Design review of the part built by this model. Coordinates are the model's own, in mm. Face numbers are marked on the shaded views. Give positions to 0.01 mm unless a question says otherwise; leave off trailing zeros. Loops run counter-clockwise (first coordinate to the right, second up) from the corner with the lowest first, then second, coordinate; pieces in that order, holes last. Notation, with made-up numbers: (-24.75, 72.5) - (2.25, 72.5) arc R20 cw to (2.25, 102.5) - close; hole circle Ø2 at (-40, -9.5). An arc over 180 degrees is marked (long way). Put each result on its own line as item: value. Start each with the question number.
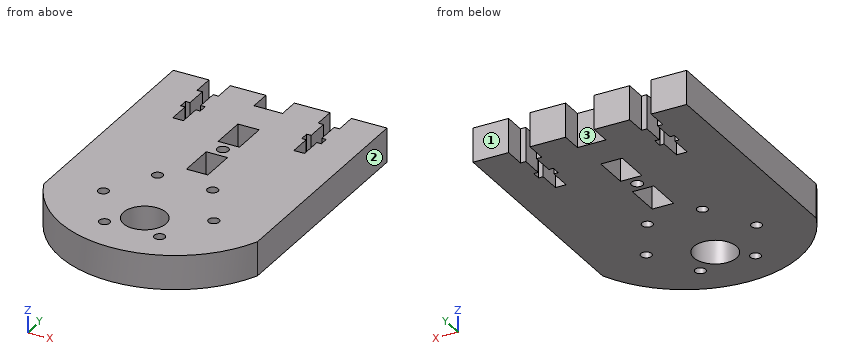
Autodesk Inventor part; units mm, degrees
ref_plane "YZ Plane" through (0, 0, 0) normal (1, 0, 0) x (0, 1, 0)
ref_plane "XZ Plane" through (0, 0, 0) normal (0, 1, 0) x (-1, 0, 0)
ref_plane "XY Plane" through (0, 0, 0) normal (0, 0, 1) x (1, 0, 0)
sketch "0" plane through (0, 0, 0) normal (0, 0, 1) x (1, 0, 0)
  line L0 (4.1594, 49.6005) -> (4.1594, 55.8505)
  line L1 (4.1594, 55.8505) -> (14.5761, 55.8505)
  line L2 (14.5761, 55.8505) -> (14.5761, 49.6005)
  line L3 (20.8261, 49.6005) -> (19.2636, 49.6005)
  line L4 (19.2636, 49.6005) -> (19.2636, 43.09)
  line L5 (19.2636, 33.9755) -> (16.1386, 33.9755)
  line L6 (16.1386, 33.9755) -> (16.1386, 40.4859)
  line L7 (14.8365, 43.09) -> (16.1386, 43.09)
  line L8 (20.5657, 43.09) -> (20.5657, 40.4859)
  line L9 (20.5657, 40.4859) -> (19.2636, 40.4859)
  line L10 (14.8365, 40.4859) -> (14.8365, 43.09)
  line L11 (16.1386, 43.09) -> (16.1386, 49.6005)
  line L12 (16.1386, 40.4859) -> (14.8365, 40.4859)
  line L13 (19.2636, 43.09) -> (20.5657, 43.09)
  line L14 (16.1386, 49.6005) -> (14.5761, 49.6005)
  line L15 (20.8261, 55.8505) -> (31.2428, 55.8505)
  line L16 (20.8261, 49.6005) -> (20.8261, 55.8505)
  line L17 (31.2428, 55.8505) -> (31.2428, 49.6005)
  line L18 (19.2636, 40.4859) -> (19.2636, 33.9755)
  line L19 (-31.2572, 49.6005) -> (-31.2572, 55.8505)
  line L20 (-31.2572, 55.8505) -> (-20.8406, 55.8505)
  line L21 (-14.5906, 55.8505) -> (-4.1739, 55.8505)
  line L22 (-4.1739, 55.8505) -> (-4.1739, 49.6005)
  line L23 (-3.1322, 49.6005) -> (-4.1739, 49.6005)
  line L24 (3.1178, 49.6005) -> (4.1594, 49.6005)
  line L25 (-20.8406, 55.8505) -> (-20.8406, 49.6005)
  line L26 (-14.5906, 49.6005) -> (-16.1531, 49.6005)
  line L27 (-16.1531, 49.6005) -> (-16.1531, 43.09)
  line L28 (-16.1531, 33.9755) -> (-19.2781, 33.9755)
  line L29 (-19.2781, 33.9755) -> (-19.2781, 40.4859)
  line L30 (-20.5802, 43.09) -> (-19.2781, 43.09)
  line L31 (-14.851, 43.09) -> (-14.851, 40.4859)
  line L32 (-14.851, 40.4859) -> (-16.1531, 40.4859)
  line L33 (-20.5802, 40.4859) -> (-20.5802, 43.09)
  line L34 (-19.2781, 43.09) -> (-19.2781, 49.6005)
  line L35 (-19.2781, 40.4859) -> (-20.5802, 40.4859)
  line L36 (-16.1531, 43.09) -> (-14.851, 43.09)
  line L37 (-19.2781, 49.6005) -> (-20.8406, 49.6005)
  line L38 (-14.5906, 49.6005) -> (-14.5906, 55.8505)
  line L39 (-16.1531, 40.4859) -> (-16.1531, 33.9755)
  arc A0 (-31.2572, -12.3787) -> (31.2428, -12.3787) centre (-0.0072, 0.6421) ccw
  circle A1 centre (8.0657, 5.7707) radius 1.5625
  circle A2 centre (-8.0802, 5.7707) radius 1.5625
  circle A3 centre (-16.1531, -8.212) radius 1.5625
  circle A4 centre (-8.0802, -22.1948) radius 1.5625
  circle A5 centre (8.0657, -22.1948) radius 1.5625
  circle A6 centre (16.1386, -8.212) radius 1.5625
  circle A7 centre (-0.0072, -15.5037) radius 6.25
  line L40 (31.2428, 49.6005) -> (31.2428, -12.3787)
  line L41 (-31.2572, -12.3787) -> (-31.2572, 49.6005)
  line L42 (-3.1322, 12.1005) -> (-3.1322, 22.5171)
  line L43 (-3.1322, 22.5171) -> (3.1178, 22.5171)
  line L44 (3.1178, 22.5171) -> (3.1178, 12.1005)
  line L45 (3.1178, 12.1005) -> (-3.1322, 12.1005)
  line L46 (-3.1322, 28.7671) -> (-3.1322, 39.1838)
  line L47 (3.1178, 39.1838) -> (3.1178, 28.7671)
  line L48 (3.1178, 28.7671) -> (-3.1322, 28.7671)
  circle A8 centre (-0.0072, 25.6421) radius 1.6667
  line L49 (-3.1322, 39.1838) -> (3.1178, 39.1838)
  line L50 (-3.1322, 49.6005) -> (3.1178, 49.6005)
  dimension "d0" = 12.5
sketch "Эскиз3" plane through (0, 0, 0) normal (0, 0, 1) x (1, 0, 0)
  circle A0 centre (-0.0072, -15.5037) radius 6.25
  circle A1 centre (-16.1531, -8.212) radius 1.5625
  circle A2 centre (-8.0802, 5.7707) radius 1.5625
  circle A3 centre (8.0657, 5.7707) radius 1.5625
  circle A4 centre (16.1386, -8.212) radius 1.5625
  circle A5 centre (8.0657, -22.1948) radius 1.5625
  circle A6 centre (-8.0802, -22.1948) radius 1.5625
  arc A7 (-31.2572, -12.3787) -> (31.2428, -12.3787) centre (-0.0072, 0.6421) ccw
  line L0 (-31.2572, -12.3787) -> (-31.2572, 49.6005)
  line L1 (-31.2572, 49.6005) -> (-31.2572, 55.8505)
  line L2 (-31.2572, 55.8505) -> (-20.8406, 55.8505)
  line L3 (-20.8406, 55.8505) -> (-20.8406, 49.6005)
  line L4 (-19.2781, 49.6005) -> (-20.8406, 49.6005)
  line L5 (-19.2781, 43.09) -> (-19.2781, 49.6005)
  line L6 (-20.5802, 43.09) -> (-19.2781, 43.09)
  line L7 (-20.5802, 40.4859) -> (-20.5802, 43.09)
  line L8 (-19.2781, 40.4859) -> (-20.5802, 40.4859)
  line L9 (-19.2781, 33.9755) -> (-19.2781, 40.4859)
  line L10 (-16.1531, 33.9755) -> (-19.2781, 33.9755)
  line L11 (-16.1531, 40.4859) -> (-16.1531, 33.9755)
  line L12 (-14.851, 40.4859) -> (-16.1531, 40.4859)
  line L13 (-14.851, 43.09) -> (-14.851, 40.4859)
  line L14 (-16.1531, 43.09) -> (-14.851, 43.09)
  line L15 (-16.1531, 49.6005) -> (-16.1531, 43.09)
  line L16 (-14.5906, 49.6005) -> (-16.1531, 49.6005)
  line L17 (-14.5906, 49.6005) -> (-14.5906, 55.8505)
  line L18 (-14.5906, 55.8505) -> (-4.1739, 55.8505)
  line L19 (-4.1739, 55.8505) -> (-4.1739, 49.6005)
  line L20 (-3.1322, 49.6005) -> (3.1178, 49.6005)
  line L21 (3.1178, 49.6005) -> (4.1594, 49.6005)
  line L22 (-3.1322, 49.6005) -> (-4.1739, 49.6005)
  line L23 (4.1594, 49.6005) -> (4.1594, 55.8505)
  line L24 (4.1594, 55.8505) -> (14.5761, 55.8505)
  line L25 (14.5761, 55.8505) -> (14.5761, 49.6005)
  line L26 (16.1386, 49.6005) -> (14.5761, 49.6005)
  line L27 (16.1386, 43.09) -> (16.1386, 49.6005)
  line L28 (14.8365, 43.09) -> (16.1386, 43.09)
  line L29 (14.8365, 40.4859) -> (14.8365, 43.09)
  line L30 (16.1386, 40.4859) -> (14.8365, 40.4859)
  line L31 (16.1386, 33.9755) -> (16.1386, 40.4859)
  line L32 (19.2636, 33.9755) -> (16.1386, 33.9755)
  line L33 (19.2636, 40.4859) -> (19.2636, 33.9755)
  line L34 (20.5657, 40.4859) -> (19.2636, 40.4859)
  line L35 (20.5657, 43.09) -> (20.5657, 40.4859)
  line L36 (19.2636, 43.09) -> (20.5657, 43.09)
  line L37 (19.2636, 49.6005) -> (19.2636, 43.09)
  line L38 (20.8261, 49.6005) -> (19.2636, 49.6005)
  line L39 (20.8261, 49.6005) -> (20.8261, 55.8505)
  line L40 (20.8261, 55.8505) -> (31.2428, 55.8505)
  line L41 (31.2428, 49.6005) -> (31.2428, -12.3787)
  line L42 (3.1178, 22.5171) -> (3.1178, 12.1005)
  circle A8 centre (-0.0072, 25.6421) radius 1.6667
  line L43 (3.1178, 28.7671) -> (-3.1322, 28.7671)
  line L44 (-3.1322, 28.7671) -> (-3.1322, 39.1838)
  line L45 (-3.1322, 39.1838) -> (3.1178, 39.1838)
  line L46 (3.1178, 39.1838) -> (3.1178, 28.7671)
  line L47 (-3.1322, 22.5171) -> (3.1178, 22.5171)
  line L48 (-3.1322, 12.1005) -> (-3.1322, 22.5171)
  line L49 (3.1178, 12.1005) -> (-3.1322, 12.1005)
  line L50 (31.2428, 55.8505) -> (31.2428, 49.6005)
  line L51 (31.2428, 55.8505) -> (31.2428, -12.3787)
  line L52 (20.8261, 55.8505) -> (31.2428, 55.8505)
  line L53 (20.8261, 55.8505) -> (20.8261, 49.6005)
  line L54 (19.2636, 49.6005) -> (20.8261, 49.6005)
  line L55 (19.2636, 43.09) -> (19.2636, 49.6005)
  line L56 (20.5657, 43.09) -> (19.2636, 43.09)
  line L57 (20.5657, 43.09) -> (20.5657, 40.4859)
  line L58 (20.5657, 40.4859) -> (19.2636, 40.4859)
  line L59 (19.2636, 40.4859) -> (19.2636, 33.9755)
  line L60 (16.1386, 33.9755) -> (19.2636, 33.9755)
  line L61 (16.1386, 40.4859) -> (16.1386, 33.8824)
  line L62 (14.8365, 40.4859) -> (16.1386, 40.4859)
  line L63 (14.8365, 43.09) -> (14.8365, 40.4859)
  line L64 (16.1386, 43.09) -> (14.8365, 43.09)
  line L65 (16.1386, 49.6005) -> (16.1386, 43.09)
  line L66 (16.1386, 49.6005) -> (14.5761, 49.6005)
  line L67 (14.5761, 49.6005) -> (14.5761, 55.8505)
  line L68 (4.1594, 55.8505) -> (14.5761, 55.8505)
  line L69 (4.1594, 55.8505) -> (4.1594, 49.6005)
  line L70 (-3.1322, 39.1838) -> (3.1178, 39.1838)
  line L71 (3.1178, 39.1838) -> (3.1178, 28.7671)
  line L72 (3.1178, 28.7671) -> (-3.1322, 28.7671)
  line L73 (-3.1322, 28.7671) -> (-3.1322, 39.1838)
  line L74 (-3.1322, 22.5171) -> (3.1178, 22.5171)
  line L75 (3.1178, 22.5171) -> (3.1178, 12.1005)
  line L76 (3.1178, 12.1005) -> (-3.1322, 12.1005)
  line L77 (-3.1322, 12.1005) -> (-3.1322, 22.5171)
  circle A9 centre (-0.0072, -15.5037) radius 6.25
  circle A10 centre (16.1386, -8.212) radius 1.5625
  circle A11 centre (8.0657, 5.7707) radius 1.5625
  circle A12 centre (8.0657, -22.1948) radius 1.5625
  circle A13 centre (-8.0802, 5.7707) radius 1.5625
  circle A14 centre (-16.1531, -8.212) radius 1.5625
  circle A15 centre (-8.0802, -22.1948) radius 1.5625
  line L78 (-14.5906, 55.8505) -> (-14.5906, 49.6005)
  line L79 (-20.8406, 49.6005) -> (-20.8406, 55.8505)
  line L80 (-14.851, 43.09) -> (-14.851, 40.4859)
  line L81 (-20.5802, 40.4859) -> (-20.5802, 43.09)
  line L82 (-16.1531, 33.9755) -> (-19.2781, 33.9755)
  line L83 (-20.8406, 55.8505) -> (-20.5802, 55.8505)
  line L84 (-14.851, 55.8505) -> (-14.5906, 55.8505)
  line L85 (-14.5906, 49.6005) -> (-16.1531, 49.6005)
  line L86 (-19.2781, 49.6005) -> (-20.8406, 49.6005)
  line L87 (-19.2781, 33.9755) -> (-19.2781, 40.4859)
  line L88 (-19.2781, 43.09) -> (-19.2781, 49.6005)
  line L89 (-16.1531, 49.6005) -> (-16.1531, 43.09)
  line L90 (-16.1531, 40.4859) -> (-16.1531, 33.9755)
  line L91 (-20.5802, 43.09) -> (-19.2781, 43.09)
  line L92 (-16.1531, 43.09) -> (-14.851, 43.09)
  line L93 (-14.851, 40.4859) -> (-16.1531, 40.4859)
  line L94 (-19.2781, 40.4859) -> (-20.5802, 40.4859)
  line L95 (-31.2572, 55.8505) -> (-31.2572, -12.3787)
  line L96 (-31.2572, 55.8505) -> (-20.5802, 55.8505)
  line L97 (-14.851, 55.8505) -> (-4.1739, 55.8505)
  line L98 (-4.1739, 55.8505) -> (-4.1739, 49.6005)
  line L99 (-4.1739, 49.6005) -> (4.1594, 49.6005)
  circle A16 centre (-0.0072, 25.6421) radius 1.6667
  arc A17 (-31.2572, -12.3787) -> (31.2428, -12.3787) centre (-0.0072, 0.6421) ccw
  point P0 (0, 0)
  point P1 (-0.0072, 12.1005)
  point P2 (3.1178, 17.3088)
  dimension "d1" = 33.8542
  dimension "d2" = 12.5
extrude "Выдавливание1" add sketch "Эскиз3" along normal blind 10
properties part number "Крепление_мотора1_платформа"
Item 1: Consider section C-C (z = 7.25). Count the separate pieces of the cut face and the enclosed holes in it, plus the area to 3 significant figures.
Item 2: For P1, Ø1, axis at x = -20, z = 5, coming from the -Y side; P2, Ø3, axis at x = 8.07, y = -22.19, coming from the -Z side; P3, Ø5, axis at x = -1.5, z = 5, coming from the -Y side; P4, Ø2, axis at y = -18, z = 2, coming from the +X side, all flat-tipped, find the tip position at first contact; note any pin that passes through.
Item 3: For L1, parallel to X at y = -8, z = 7.5; L2, parallel to X at y = 37.5, z = 7; L3, parallel to Y at x = -0.5, z = 2, list the stretches that pass through material, from the lowest coordinate up. Write a range as from..to.
Item 4: Consider section A-A (y = 17.5). State the section outline as (x, z) points, plus the area to 4 significant figures.
Item 5: Mouldability with a two-part tool opening along X and no side actions: class the marked faces 1, 2 and 3 as pulls with the +X half, pulls with the -X half, needs draft (parallel to the pull), parting line crosses it, or undercut.
Item 6: Consider section B-B (x = -8). State the section outline as (y, z) points (1 decimal), plus the area to 3 significant figures.
Item 7: Consider section D-D (y = -18.5). State the section outline as (x, z) points, plus the area to 3 significant figures.
Geometry says:
1. separate pieces: 1
1. enclosed holes: 10
1. area: 4,660 mm2
2. P1: stops at y = -27.04
2. P2: passes through
2. P3: stops at y = -33.21
2. P4: stops at x = 28.89
3. L1: x = -31.26..-17.7, -14.61..14.59, 17.69..31.24
3. L2: x = -31.26..-19.28, -16.15..-3.13, 3.12..16.14, 19.26..31.24
3. L3: y = -33.21..-21.73, -9.27..12.1, 22.52..24.05, 27.23..28.77, 39.18..49.6
4. outline: (-31.26, 0) - (-3.13, 0) - (-3.13, 10) - (-31.26, 10) - close; (3.12, 0) - (31.24, 0) - (31.24, 10) - (3.12, 10) - close
4. area: 562.5 mm2
5. face 1: needs draft
5. face 2: pulls with the +X half
5. face 3: undercut
6. outline: (-32.3, 0) - (-23.8, 0) - (-23.8, 10) - (-32.3, 10) - close; (-20.6, 0) - (4.2, 0) - (4.2, 10) - (-20.6, 10) - close; (7.3, 0) - (55.9, 0) - (55.9, 10) - (7.3, 10) - close
6. area: 819 mm2
7. outline: (-27.93, 0) - (-5.49, 0) - (-5.49, 10) - (-27.93, 10) - close; (5.48, 0) - (27.92, 0) - (27.92, 10) - (5.48, 10) - close
7. area: 449 mm2
